Read the model definition and answer for the solid it produces. Units are mm, in the model's axes. Face numbers are marked on the shaded views. A direction names the side the tool comes from. Coordinates: 2 decimals unless noted, no trailing zeros. Write each loop counter-clockwise with the first axis right and the second up, starting at its lowest first coordinate (ties: lowest second). Pieces come first, ordered by that corner, then holes.
(1) The part is cut by section A-A, the plane y = 5. Determine the outline of the cut face in (x, z), and give its area (3 significant figures).
(2) Given pin 1 (5 mm diameter, centred on x = 23, y = -7, fed in from -Z), flat-ended and moving along its own axis, determine where the tip first touches the part or whether it passes through.
(3) The part is cut by section B-B, the plane x = 0. Determine the outline of the cut face in (y, z).
(4) The part is cut by section D-D, the plane x = 17. Determine the outline of the cut face in (y, z), and give its area (3 significant figures).
(5) Straight lines are drawn through the part: line 1 along Y through (x, z) = (37.5, 0.95); line 2 along Y through (x, z) = (0, 1.15); line 3 along X through (y, z) = (-1.25, 1.85). For each, find the intervals that lie inside material, in ascending order.
(6) Which of the six approach directions +Z, -Z, +X, -X, +Y, -Y give full straight-line access (tool end or side, diameter ignored) to the marked faces 1, 2 and 3?
(7) The part is cut by section C-C, the plane z = 0.75. State how many separate pieces and enclosed holes the cut face has, and give its area (3 significant figures).
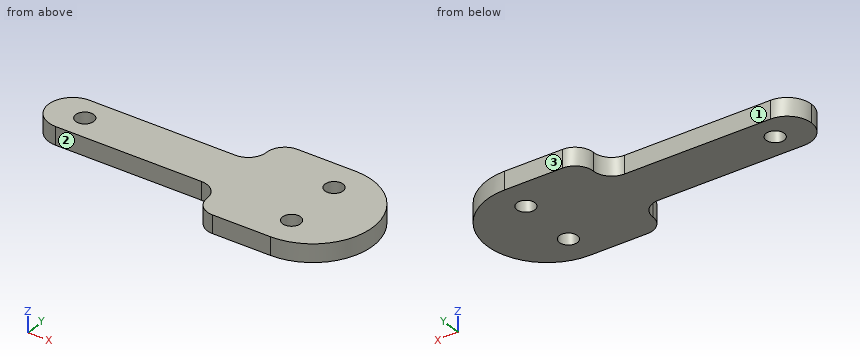
Autodesk Inventor part; units mm, degrees
ref_plane "YZ Plane" through (0, 0, 0) normal (1, 0, 0) x (0, 1, 0)
ref_plane "XZ Plane" through (0, 0, 0) normal (0, 1, 0) x (-1, 0, 0)
ref_plane "XY Plane" through (0, 0, 0) normal (0, 0, 1) x (1, 0, 0)
sketch "Sketch1" plane through (0, 0, 0) normal (0, 0, 1) x (1, 0, 0)
  line L0 (0, 0) -> (37.5, 0) construction
  line L1 (0, -10) -> (37.5, -10)
  line L2 (37.5, 10) -> (0, 10)
  arc A0 (0, 10) -> (0, -10) centre (0, 0) ccw
  arc A1 (37.5, -10) -> (37.5, 10) centre (37.5, 0) ccw
  line L3 (0, 0) -> (37.5, 0) construction
  circle A2 centre (0, 0) radius 1.5
  circle A3 centre (37.5, -5) radius 1.5
  circle A4 centre (37.5, 5) radius 1.5
  point P0 (18.75, 0)
  dimension "d0" = 37.5
  dimension "d1" = 0
  dimension "d2" = 20
  dimension "d3" = 3
  dimension "d4" = 3
  dimension "d5" = 3
  dimension "d6" = 10
  dimension "d7" = 5
  dimension "d8" = 0
  dimension "d9" = 0
extrude "Extrusion1" add sketch "Sketch1" along normal blind 3
sketch "Sketch2" plane through (0, 0, 0) normal (0, 0, -1) x (-1, 0, 0)
  line L0 (6, 4) -> (-25, 4)
  line L1 (-25, 10) -> (-25, -10)
  line L2 (-25, -4) -> (6, -4)
  line L3 (6, -4) -> (6, 4)
  arc A0 (-37.5, 10) -> (-37.5, -10) centre (-37.5, 0) ccw
  line L4 (0, -10) -> (-37.5, -10)
  arc A1 (0, -10) -> (0, 10) centre (0, 0) ccw
  line L5 (-37.5, 10) -> (0, 10)
  circle A2 centre (-37.5, 5) radius 1.5
  circle A3 centre (-37.5, -5) radius 1.5
  circle A4 centre (0, 0) radius 1.5
  dimension "d12" = 6
  dimension "d13" = 4
  dimension "d14" = 4
  dimension "d15" = 25
extrude "Extrusion2" cut sketch "Sketch2" against normal up to surface (3 mm away) contours L0 L1 L5 A1 L4 L2 L3
fillet "Fillet1" radius 3 4 edges at (25, 4, 1.5) (25, 10, 1.5) (25, -4, 1.5) (25, -10, 1.5)
fillet "Fillet2" radius 4 2 edges at (-6, 4, 1.5) (-6, -4, 1.5)
properties part number "Arm5" material "Aluminum 6061, Welded"
Computed:
1. outline: (24.24, 0) - (36, 0) - (36, 3) - (24.24, 3) - close; (39, 0) - (46.16, 0) - (46.16, 3) - (39, 3) - close
1. area: 56.8 mm2
2. pin 1: stops at z = 0
3. outline: (-4, 0) - (-1.5, 0) - (-1.5, 3) - (-4, 3) - close; (1.5, 0) - (4, 0) - (4, 3) - (1.5, 3) - close
4. outline: (-4, 0) - (4, 0) - (4, 3) - (-4, 3) - close
4. area: 24.0 mm2
5. line 1: y = -10 to -6.5, -3.5 to 3.5, 6.5 to 10
5. line 2: y = -4 to -1.5, 1.5 to 4
5. line 3: x = -5.8 to -0.83, 0.83 to 47.42
6. face 1: +Z, -Z, -X, +Y
6. face 2: +Z, -Z, -X, -Y
6. face 3: +Z, -Z, +X, -X, +Y
7. separate pieces: 1
7. enclosed holes: 3
7. area: 627 mm2
